Input: part model. Units: mm. Frame: model coordinates. A direction names the side the tool comes from. Coordinates: 2 decimals unless noted, no trailing zeros. Loops run counter-clockwise (first coordinate to the right, second up) from the corner with the lowest first, then second, coordinate; pieces in that order, holes last.
(1) Line query: L1, parallel to Y at x = 8, z = -22.5; L2, parallel to X at y = 2, z = -4; L3, parallel to Y at x = 60, z = -20. Output: solid intervals per line, ascending.
(2) Section B-B, the plane z = -42. Return loops of the section in (x, y), then the cut area to 3 significant figures.
(3) Set-up query: faces 4 (the face through (-8.23, 41.71, -17.79)), 5 (the face through (25, 4, -40)), 6 (the face through (15.8, 23, -20)). Return all of +Z, -Z, +X, -X, +Y, -Y with unobstructed straight access to the full face (end or side cutting, diameter ignored); none if empty.
(4) Section A-A, the plane x = -102. Return loops of the section in (y, z), then the cut area to 3 significant figures.
(5) Mould query, pull axis Z, two halves, no side actions, for faces 1 (the face through (33.32, 34.88, -36.3)), 2 (the face through (35, 28, -48.1)), 3 (the face through (0, 4, -20)). Classes: released by +Z, released by -Z, zero draft, split by the parting line, or undercut.
(6) Contact query for flat-ended pins moving along their axis: P1, Ø10, axis at x = -29.5, z = -29, coming from the +Y side; P2, Ø2, axis at x = 34.4, y = 30, coming from the +Z side; P3, Ø5, axis at y = 29.5, z = -22, coming from the -X side; P4, Ø6, axis at x = 10.5, z = -27, coming from the -Y side. Output: stop coordinate, or through.
```python
from build123d import *

# Parameters (mm, degrees)
BOSS_EXTRUDE1_DEPTH  = 8.2
SKETCH2_W            = 25.2
SKETCH2_H            = 25.2
BOSS_EXTRUDE2_DEPTH  = 32.5
SKETCH3_W            = 25.2
SKETCH3_H            = 9.6
BOSS_EXTRUDE3_DEPTH  = 6
SKETCH4_W            = 25.2
SKETCH4_H            = 25.2
BOSS_EXTRUDE4_DEPTH  = 30
CHAMFER1_SIZE        = 7
SKETCH5_R            = 5
BOSS_EXTRUDE5_DEPTH  = 7.5
SKETCH6_R            = 9
BOSS_EXTRUDE6_DEPTH  = 8
SKETCH7_R            = 1.25
CUT_EXTRUDE1_DEPTH   = 4
SKETCH8_R            = 5
BOSS_EXTRUDE7_DEPTH  = 7.5
SKETCH9_R            = 9
BOSS_EXTRUDE8_DEPTH  = 8
SKETCH10_R           = 1.25
CUT_EXTRUDE2_DEPTH   = 4
SKETCH11_R           = 5
BOSS_EXTRUDE9_DEPTH  = 7.5
SKETCH12_R           = 9
BOSS_EXTRUDE10_DEPTH = 8
SKETCH13_R           = 1.25
CUT_EXTRUDE3_DEPTH   = 4
SKETCH15_R           = 3
CUT_EXTRUDE4_REACH   = 139.748
SKETCH16_R           = 1.5


with BuildPart() as part:
    # Sketch1 → Boss-Extrude1 (new body)
    with BuildSketch(Plane(origin=(0, 0, 0), x_dir=(1, 0, 0), z_dir=(0, 1, 0))):
        with BuildLine():
            Line((2, 0), (48, 0))
            ThreePointArc((48, 0), (49.414213562, 0.585786438), (50, 2))
            Line((50, 2), (50, 38))
            ThreePointArc((50, 38), (49.414213562, 39.414213562), (48, 40))
            Line((48, 40), (2, 40))
            ThreePointArc((2, 40), (0.585786438, 39.414213562), (0, 38))
            Line((0, 38), (0, 2))
            ThreePointArc((0, 2), (0.585786438, 0.585786438), (2, 0))
        make_face()
    extrude(amount=BOSS_EXTRUDE1_DEPTH)

    # Sketch2 → Boss-Extrude2 (add)
    with BuildSketch(Plane(origin=(0, 8.2, 0), x_dir=(1, 0, 0), z_dir=(0, 1, 0))):
        with Locations((34.4, 20)):
            Rectangle(SKETCH2_W, SKETCH2_H)
    extrude(amount=BOSS_EXTRUDE2_DEPTH)

    # Sketch3 → Boss-Extrude3 (add)
    with BuildSketch(Plane.ZY.offset(-21.8)):
        with Locations((-20, 35.9)):
            Rectangle(SKETCH3_W, SKETCH3_H)
    extrude(amount=BOSS_EXTRUDE3_DEPTH)

    # Sketch4 → Boss-Extrude4 (add)
    with BuildSketch(Plane.ZY.offset(-15.8)):
        with Locations((-20, 28.1)):
            Rectangle(SKETCH4_W, SKETCH4_H)
    extrude(amount=BOSS_EXTRUDE4_DEPTH)

    # Chamfer1
    chamfer1_edges = [part.edges().sort_by_distance(p)[0] for p in [
        (-14.2, 28.1, -32.6),
        (-14.2, 28.1, -7.4),
    ]]
    chamfer(chamfer1_edges, length=CHAMFER1_SIZE)

    # Sketch5 → Boss-Extrude5 (add)
    with BuildSketch(Plane(origin=(47, 0, 0), x_dir=(0, 0, -1), z_dir=(1, 0, 0))):
        with Locations(Location((20, 16, 0), (0, 0, 180))):
            Circle(SKETCH5_R)
    extrude(amount=BOSS_EXTRUDE5_DEPTH)

    # Sketch6 → Boss-Extrude6 (add)
    with BuildSketch(Plane(origin=(54.5, 0, 0), x_dir=(0, 0, -1), z_dir=(1, 0, 0))):
        with Locations((20, 16)):
            Circle(SKETCH6_R)
    extrude(amount=BOSS_EXTRUDE6_DEPTH)

    # Sketch7 → Cut-Extrude1 (cut)
    with BuildSketch(Plane(origin=(62.5, 0, 0), x_dir=(0, 0, -1), z_dir=(1, 0, 0))):
        with Locations((20, 16)):
            Circle(SKETCH7_R)
    extrude(amount=-CUT_EXTRUDE1_DEPTH, mode=Mode.SUBTRACT)

    # Sketch8 → Boss-Extrude7 (add)
    with BuildSketch(Plane(origin=(0, 0, -32.6), x_dir=(-1, 0, 0), z_dir=(0, 0, -1))):
        with Locations(Location((-34.4, 30, 0), (0, 0, 180))):
            Circle(SKETCH8_R)
    extrude(amount=BOSS_EXTRUDE7_DEPTH)

    # Sketch9 → Boss-Extrude8 (add)
    with BuildSketch(Plane(origin=(0, 0, -40.1), x_dir=(-1, 0, 0), z_dir=(0, 0, -1))):
        with Locations((-34.4, 30)):
            Circle(SKETCH9_R)
    extrude(amount=BOSS_EXTRUDE8_DEPTH)

    # Sketch10 → Cut-Extrude2 (cut)
    with BuildSketch(Plane(origin=(0, 0, -48.1), x_dir=(-1, 0, 0), z_dir=(0, 0, -1))):
        with Locations((-34.4, 30)):
            Circle(SKETCH10_R)
    extrude(amount=-CUT_EXTRUDE2_DEPTH, mode=Mode.SUBTRACT)

    # Sketch11 → Boss-Extrude9 (add)
    with BuildSketch(Plane(origin=(0, 40.7, 0), x_dir=(1, 0, 0), z_dir=(0, 1, 0))):
        with Locations(Location((7, 20, 0), (0, 0, 270))):
            Circle(SKETCH11_R)
    extrude(amount=BOSS_EXTRUDE9_DEPTH)

    # Sketch12 → Boss-Extrude10 (add)
    with BuildSketch(Plane(origin=(0, 48.2, 0), x_dir=(1, 0, 0), z_dir=(0, 1, 0))):
        with Locations(Location((7, 20, 0), (0, 0, 270))):
            Circle(SKETCH12_R)
    extrude(amount=BOSS_EXTRUDE10_DEPTH)

    # Sketch13 → Cut-Extrude3 (cut)
    with BuildSketch(Plane(origin=(0, 56.2, 0), x_dir=(1, 0, 0), z_dir=(0, 1, 0))):
        with Locations(Location((7, 20, 0), (0, 0, 270))):
            Circle(SKETCH13_R)
    extrude(amount=-CUT_EXTRUDE3_DEPTH, mode=Mode.SUBTRACT)

    # Sweep1: sweep along a path in Sketch14
    with BuildLine(Plane.XY.offset(-20)) as sweep1_path:
        Line((-6.2, 40.7), (-6.2, 42.7))
        ThreePointArc((-6.2, 42.7), (-7.459440841, 45.740559159), (-10.5, 47))
        Line((-10.5, 47), (-116.2, 47))
    # Sketch15 → Sweep1 (sweep)
    with BuildSketch(Plane(origin=(-116.2, 0, 0), x_dir=(0, 0, -1), z_dir=(1, 0, 0))):
        with Locations((20, 47)):
            Circle(SKETCH15_R)
    sweep(path=sweep1_path.line)

    # Sketch16 → Cut-Extrude4 (cut, up to next)
    with BuildSketch(Plane.XZ, mode=Mode.PRIVATE) as cut_extrude4_sk1:
        with Locations(Location((41, -4, 0), (0, 0, 270))):
            Circle(SKETCH16_R)
    cut_extrude4_tool1 = extrude(cut_extrude4_sk1.sketch, amount=-CUT_EXTRUDE4_REACH, mode=Mode.PRIVATE) & part.part
    # Sketch16 → Cut-Extrude4 (cut, up to next)
    with BuildSketch(Plane.XZ, mode=Mode.PRIVATE) as cut_extrude4_sk2:
        with Locations(Location((41, -36, 0), (0, 0, 270))):
            Circle(SKETCH16_R)
    cut_extrude4_tool2 = extrude(cut_extrude4_sk2.sketch, amount=-CUT_EXTRUDE4_REACH, mode=Mode.PRIVATE) & part.part
    add(cut_extrude4_tool1.solids().sort_by_distance((41, 0, -4))[0], mode=Mode.SUBTRACT)
    add(cut_extrude4_tool2.solids().sort_by_distance((41, 0, -36))[0], mode=Mode.SUBTRACT)


solid = part.part
```
Report:
1. L1: y = 0 to 8.2, 15.5 to 56.2
1. L2: x = 0 to 39.5, 42.5 to 50
1. L3: y = 7 to 14.75, 17.25 to 25
2. outline: circle Ø18 at (34.4, 30)
2. area: 254 mm2
3. face 4: none
3. face 5: -Z, +X, -X, -Y
3. face 6: +Z, -Z
4. outline: circle Ø6 at (47, -20)
4. area: 28.3 mm2
5. face 1: undercut
5. face 2: released by -Z
5. face 3: zero draft
6. P1: passes through
6. P2: stops at z = -7.4
6. P3: stops at x = -14.2
6. P4: stops at y = 0
